Source: CAD feature listing. Evaluate the final solid. Frame: model axes, mm. A direction names the side the tool comes from. Give positions to 0.01 mm unless a question says otherwise; leave off trailing zeros. Order: outer loops, then holes, each group sorted by start corner. A loop starts at its lowest first (then second) coordinate and runs counter-clockwise, first axis right, second up.
```python
from build123d import *

# Parameters (mm, degrees)
F2_R            = 12.1598954619
F3_DEPTH        = 16
F5_DEPTH        = 16
F5_COPIES_COUNT = 16
F8_R            = 14.6598954619
F8_R_2          = 12.1598954619
F9_DEPTH        = 1.5
F10_DEPTH       = 17.501


# Not quite as in the source:
# - a feature of the source that left no trace in its solid (it failed there, or was rolled back) is left out
# - a pattern or mirror of a feature is missing from the dataset's text; its kind, count and spacing are read off the source's solid


with BuildPart() as f3:
    # F2 (on Top) → F3 (new body)
    with BuildSketch(Plane.XY):
        Circle(F2_R)
    extrude(amount=F3_DEPTH)

    # F4 (on face) → F5 (cut, through all)
    with BuildSketch(Plane.XY.offset(16)):
        with BuildLine():
            ThreePointArc((-2.024177758, 11.9902361131), (-1.6634915573, 11.8941223999), (-1.4994378615, 11.5588333213))
            ThreePointArc((-1.4994378615, 11.5588333213), (0, 10.0998954619), (1.4994378615, 11.5588333213))
            ThreePointArc((1.4994378615, 11.5588333213), (1.6634915573, 11.8941223999), (2.024177758, 11.9902361131))
            ThreePointArc((2.024177758, 11.9902361131), (0, 12.1598954619), (-2.024177758, 11.9902361131))
        make_face()
    f5 = extrude(amount=-F5_DEPTH, mode=Mode.SUBTRACT)

    # F5_copies: F5 ×16 about axis
    f5_copies_axis = Axis((0, 0, 0), (0, 0, 1))
    for i in range(1, F5_COPIES_COUNT):
        add(f5.rotate(f5_copies_axis, i * 360 / F5_COPIES_COUNT), mode=Mode.SUBTRACT)

    # F8 (on face) + F2 (on Top) → F9 (join)
    with BuildSketch(Plane.XY):
        Circle(F8_R)
        Circle(F8_R_2, mode=Mode.SUBTRACT)
    with BuildSketch(Plane.XY):
        Circle(F2_R)
    extrude(amount=-F9_DEPTH)

    # F7 (on face) → F10 (cut, through all)
    with BuildSketch(Plane.XY.offset(16)):
        Polygon((3.7527767497, 6.5), (-3.7527767497, 6.5), (-7.5055534995, 0), (-3.7527767497, -6.5), (3.7527767497, -6.5), (7.5055534995, 0), align=None)
    extrude(amount=-F10_DEPTH, mode=Mode.SUBTRACT)


solid = f3.part
```
1) Material intervals for L1, parallel to X at y = -7, z = 14; L2, parallel to Y at x = -0.25, z = 2.5; L3, parallel to X at y = 2.5, z = 12.5, sorted ascending.
Report:
L1: x = -9.94 to -9.1, -7.31 to 7.31, 9.1 to 9.94
L2: y = -10.12 to -6.5, 6.5 to 10.12
L3: x = -11.9 to -6.06, 6.06 to 11.9
2) Section query A-A, the plane x = 0. Return the cut outline in (y, z), and give its area (3 significant figures).
Report:
outline: (-14.66, -1.5) - (-6.5, -1.5) - (-6.5, 16) - (-10.1, 16) - (-10.1, 0) - (-14.66, 0) - close; (6.5, -1.5) - (14.66, -1.5) - (14.66, 0) - (10.1, 0) - (10.1, 16) - (6.5, 16) - close
area: 140 mm2
3) Pin query (flat end, axial travel): pin 1 (1.5 mm diameter, centred on y = -2.5, z = 3, fed in from +X); pin 2 (5 mm diameter, centred on x = 3.5, z = 12, fed in from +Y); pin 3 (2 mm diameter, centred on x = 11.5, z = 11.5, fed in from +Y). Return the tip coordinate at first contact, or that it passes through.
Report:
pin 1: stops at x = 12
pin 2: stops at y = 12
pin 3: stops at y = 3.07
4) Reachability of faces 4 (the cylindrical face through (-7.119, -7.165, 8.112)), 5 (the cylindrical face through (10.1, 0, 8.1)), 6 (the flat face through (0, 6.5, 7)) from +Z, -Z, +X, -X, +Y, -Y: full face, straight path, thin tool, end or side. Return the list, or none.
Report:
face 4: +Z
face 5: +Z, +X
face 6: +Z, -Z
5) Section query B-B, the plane y = -3.5. Return the cut outline in (x, z), and give its area (3 significant figures).
Report:
outline: (-14.24, -1.5) - (-5.48, -1.5) - (-5.48, 16) - (-9.55, 16) - (-9.55, 0) - (-14.24, 0) - close; (5.48, -1.5) - (14.24, -1.5) - (14.24, 0) - (9.55, 0) - (9.55, 16) - (5.48, 16) - close
area: 156 mm2
6) Section query C-C, the plane x = 8.25. Return the cut outline in (y, z), and give its area (3 significant figures).
Report:
outline: (-12.12, -1.5) - (12.12, -1.5) - (12.12, 0) - (6.7, 0) - (6.7, 16) - (-6.7, 16) - (-6.7, 0) - (-12.12, 0) - close
area: 251 mm2
7) Draft query along Y for faces 1 (the cylindrical face through (0, 10.1, 8.1)), 2 (the cylindrical face through (7.165, -7.119, 8.112)), 3 (the flat face through (5, -5, 16)). Return one class per face: +Y half, -Y half, draft (parallel to the pull), parting line (faces both ways), or undercut.
Report:
face 1: +Y half
face 2: undercut
face 3: draft
